Geometry: see drawing. Coordinates: mm, zero at the bounding-box minimum. A direction names the side the tool comes from. Give positions to 0.01 mm unless a question says otherwise; leave off trailing zeros. Loops run counter-clockwise (first coordinate to the right, second up) from the corner with the lowest first, then second, coordinate; pieces in that order, holes last. Notation, with made-up numbers: (-3.75, 33.5) -> (52.25, 33.5) arc R16 ccw to (52.25, 52.5) -> close; hole circle Ø9 at (51, 3). An arc over 180 degrees is marked (long way). Return JSON: item names as keys, results as strings. Group by question number.
(1) Cut plane C-C on z = 15.5. Return loops of the section in (x, y).
(2) Ray query, line 1 (Z direction, x = 100, y = 30) (3 decimals); line 2 (X direction, y = 30.5, z = 42.5); line 3 (Z direction, x = 169.5, y = 14.5) (3 decimals). Return the intervals inside material, ascending. Write a range as from..to.
(3) Cut plane A-A on y = 36. Return loops of the section in (x, z) (3 decimals), then the cut area to 3 significant figures.
(4) Pin query (flat end, axial travel): pin 1 (4 mm diameter, centred on x = 27.5, y = 49, fed in from -Z) (3 decimals); pin 2 (3 mm diameter, centred on y = 26, z = 128, fed in from -X); pin 3 (22 mm diameter, centred on y = 35, z = 93.5, fed in from +X). Return the tip coordinate at first contact, or that it passes through.
(5) Access query for the marked faces 1, 2, 3 and 4. Directions: +Z, -Z, +X, -X, +Y, -Y. A direction counts if a zero-diameter tool reaches every point of the face in a straight line with its end or side. Return the directions, or none.
(6) Cut plane B-B on x = 37.5. Return loops of the section in (y, z) (3 decimals).
(7) Draft query along Z for the marked faces 5, 6 and 7. Return one class per face: released by +Z, released by -Z, zero draft, split by the parting line, or undercut.
(8) Cut plane D-D on y = 22.5. Return loops of the section in (x, z) (3 decimals), then the cut area to 3 significant figures.
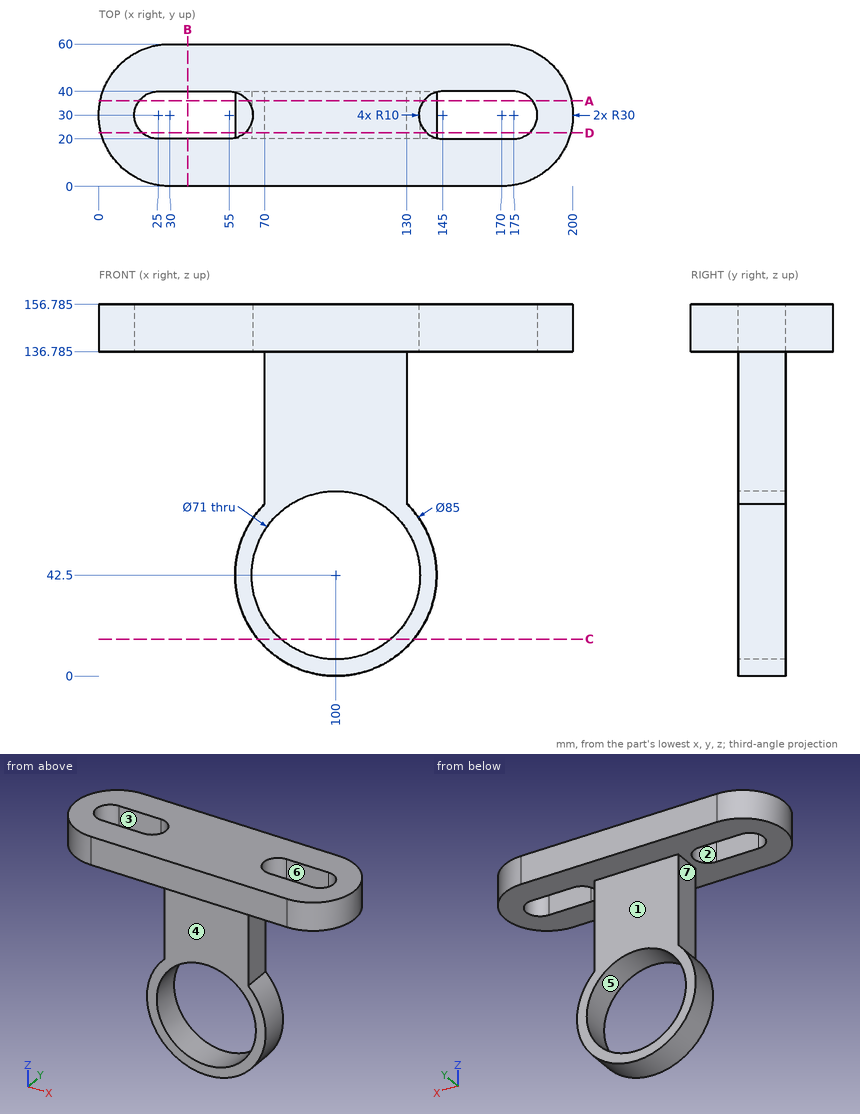
Answers:
{
 "1": {"outline": "(67.18, 20) -> (76.95, 20) -> (76.95, 40) -> (67.18, 40) -> close; (123.05, 20) -> (132.82, 20) -> (132.82, 40) -> (123.05, 40) -> close"},
 "2": {"line 1": "0..7, 78..156.785", "line 2": "57.5..64.5, 135.5..142.5", "line 3": "136.785..156.785"},
 "3": {"outline": "(0.606, 136.785) -> (17, 136.785) -> (17, 156.785) -> (0.606, 156.785) -> close; (63, 136.785) -> (70, 136.785) -> (70, 72.604) arc R42.5 ccw (long way) to (130, 72.604) -> (130, 136.785) -> (137, 136.785) -> (137, 156.785) -> (63, 156.785) -> close; (183, 136.785) -> (199.394, 136.785) -> (199.394, 156.785) -> (183, 156.785) -> close; hole circle Ø71 at (100, 42.5)", "area": "7,190 mm²"},
 "4": {"pin 1": "z = 136.785", "pin 2": "x = 70", "pin 3": "x = 130"},
 "5": {"face 1": "-Z, +X, -X, +Y", "face 2": "+Z", "face 3": "+Z, -Z", "face 4": "-Z, +X, -X, -Y"},
 "6": {"outline": "(0, 136.785) -> (20, 136.785) -> (20, 156.785) -> (0, 156.785) -> close; (40, 136.785) -> (60, 136.785) -> (60, 156.785) -> (40, 156.785) -> close"},
 "7": {"face 5": "undercut", "face 6": "zero draft", "face 7": "undercut"},
 "8": {"outline": "(0.953, 136.785) -> (18.386, 136.785) -> (18.386, 156.785) -> (0.953, 156.785) -> close; (61.614, 136.785) -> (70, 136.785) -> (70, 72.604) arc R42.5 ccw (long way) to (130, 72.604) -> (130, 136.785) -> (138.386, 136.785) -> (138.386, 156.785) -> (61.614, 156.785) -> close; (181.614, 136.785) -> (199.047, 136.785) -> (199.047, 156.785) -> (181.614, 156.785) -> close; hole circle Ø71 at (100, 42.5)", "area": "7,290 mm²"}
}
